```python
from build123d import *

# Parameters (mm, degrees)
SKETCH1_W                   = 33
SKETCH1_H                   = 30
BOSS_EXTRUDE1_DEPTH         = 10
CUT_EXTRUDE1_REACH          = 12
SKETCH2_R                   = 7
SKETCH3_R                   = 14.5
CUT_EXTRUDE2_DEPTH          = 8
TAP_DRILL_FOR_M3_TAP2_D     = 2.5
TAP_DRILL_FOR_M3_TAP2_DEPTH = 8
TAP_DRILL_FOR_M3_TAP2_TIP   = 0.751075774


with BuildPart() as part:
    # Sketch1 → Boss-Extrude1 (new body)
    with BuildSketch(Plane.XY):
        with Locations((16.5, 15)):
            Rectangle(SKETCH1_W, SKETCH1_H)
    extrude(amount=BOSS_EXTRUDE1_DEPTH)

    # Sketch2 → Cut-Extrude1 (cut, up to next)
    with BuildSketch(Plane.XY.offset(10), mode=Mode.PRIVATE) as cut_extrude1_sk1:
        with Locations((16.5, 15)):
            Circle(SKETCH2_R)
    cut_extrude1_tool1 = extrude(cut_extrude1_sk1.sketch, amount=-CUT_EXTRUDE1_REACH, mode=Mode.PRIVATE) & part.part
    add(cut_extrude1_tool1.solids().sort_by_distance((16.5, 15, 10))[0], mode=Mode.SUBTRACT)

    # Sketch3 → Cut-Extrude2 (cut)
    with BuildSketch(Plane(origin=(0, 0, 0), x_dir=(-1, 0, 0), z_dir=(0, 0, -1))):
        with Locations((-16.5, 15)):
            Circle(SKETCH3_R)
    extrude(amount=-CUT_EXTRUDE2_DEPTH, mode=Mode.SUBTRACT)

    # Tap Drill for M3 Tap2
    with Locations(Plane(origin=(0, 0, 0), x_dir=(-1, 0, 0), z_dir=(0, -1, 0))):
        with Locations((-3, -6), (-30, -6)):
            Hole(TAP_DRILL_FOR_M3_TAP2_D / 2, depth=TAP_DRILL_FOR_M3_TAP2_DEPTH)
            with Locations((0, 0, -(TAP_DRILL_FOR_M3_TAP2_DEPTH + TAP_DRILL_FOR_M3_TAP2_TIP / 2))):  # 118° drill point
                Cone(0, TAP_DRILL_FOR_M3_TAP2_D / 2, TAP_DRILL_FOR_M3_TAP2_TIP, mode=Mode.SUBTRACT)


solid = part.part
```
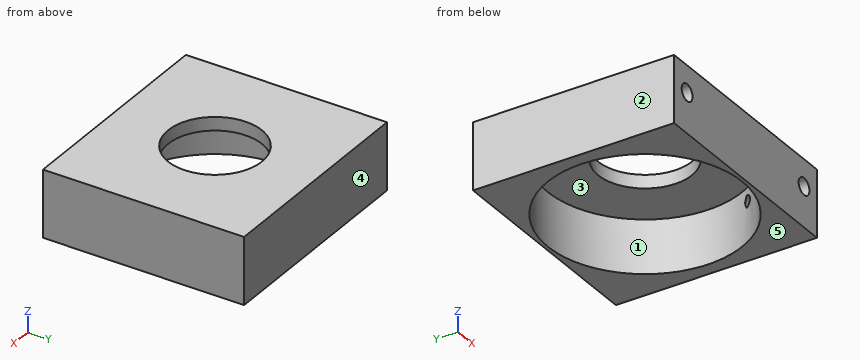
Here's how the part is built. I have some questions about the finished solid (model axes, mm). Face numbers are marked on the shaded views. A direction names the side the tool comes from. Coordinates: 2 decimals unless noted, no trailing zeros. Order: outer loops, then holes, each group sorted by start corner. A loop starts at its lowest first (then second) coordinate and runs counter-clockwise, first axis right, second up.
Item 1: If we section it at C-C, the plane z = 2.75: List the corners of the cut face in (x, y) for me.
Response values:
outline: (0, 0) - (33, 0) - (33, 30) - (0, 30) - close; hole circle Ø29 at (16.5, 15)
Item 2: Which directions (+Z, -Z, +X, -X, +Y, -Y) give clear straight access to the entire face, cutting with the end or side of a thin tool? Please do the marked faces 1 and 2.
Response values:
face 1: -Z
face 2: +Z, -Z, -X, +Y, -Y
Item 3: I'm going to push flat-ended pins straight in: pin 1 Ø6 at (x, y) = (18.5, 15) entering from -Z; pin 2 Ø1 at (x, y) = (28.5, 21) entering from -Z. Where does each tip first touch, or does it pass through?
Response values:
pin 1: passes through
pin 2: stops at z = 8
Item 4: Thinking about a two-plate mould opening in Y: for the marked faces 3, 4 and 5, which applies, pulls with the +Y half, pulls with the -Y half, needs draft (parallel to the pull), parting line crosses it, or undercut?
Response values:
face 3: undercut
face 4: pulls with the +Y half
face 5: needs draft
Item 5: If we section it at A-A, the plane x = 16.5: List the corners of the cut face in (y, z) for me, then the cut area to 3 significant figures.
Response values:
outline: (0, 0) - (0.5, 0) - (0.5, 8) - (8, 8) - (8, 10) - (0, 10) - close; (22, 8) - (29.5, 8) - (29.5, 0) - (30, 0) - (30, 10) - (22, 10) - close
area: 40.0 mm2
Item 6: If we section it at D-D, the plane x = 28: List the corners of the cut face in (y, z) for me, then the cut area to 3 significant figures.
Response values:
outline: (0, 0) - (6.17, 0) - (6.17, 8) - (23.83, 8) - (23.83, 0) - (30, 0) - (30, 10) - (0, 10) - close
area: 159 mm2
Item 7: I need wall thicknesses on probe 1 along X at (y, z) = (15.5, 6); probe 2 along Y at (x, z) = (16.5, 2.25); probe 3 along X at (y, z) = (22, 6.5). Which ranges of each line are inside material? Lowest first, please.
Response values:
probe 1: x = 0 to 2.01, 30.99 to 33
probe 2: y = 0 to 0.5, 29.5 to 30
probe 3: x = 0 to 3.8, 29.2 to 33
Item 8: If we section it at B-B, the plane y = 15: List the corners of the cut face in (x, z) for me.
Response values:
outline: (0, 0) - (2, 0) - (2, 8) - (9.5, 8) - (9.5, 10) - (0, 10) - close; (23.5, 8) - (31, 8) - (31, 0) - (33, 0) - (33, 10) - (23.5, 10) - close
